The listing builds one solid part. Answer for the finished solid, in the listing's coordinates (mm). Face numbers are marked on the shaded views. Round coordinates to 2 decimals unless told otherwise and drop trailing zeros. Write each loop counter-clockwise with the first axis right and the second up, starting at its lowest first coordinate (ties: lowest second). Pieces come first, ordered by that corner, then holes. Notation, with made-up numbers: (36, 15) - (44, 15) arc R27 cw to (44, 39) - close; hole circle Ø11 at (21, -18). An arc over 180 degrees is marked (long way). Use a Markdown table: item, result. Add a question column.
1) A cutting plane is placed at B-B (x = 63.5). Give the vertices of the cut face in (y, z), then the cut area to 3 significant figures.
2) A cutting plane is placed at D-D (y = 26.5). Give the vertices of the cut face in (x, z), then the cut area to 3 significant figures.
3) A cutting plane is placed at C-C (z = -2). Give the vertices of the cut face in (x, y), then the cut area to 3 significant figures.
4) A cutting plane is placed at A-A (y = 42). Give the vertices of the cut face in (x, z), then the cut area to 3 significant figures.
5) Determine the mould class of the marked faces 1, 2 and 3 for opening direction X: +X half, -X half, draft (parallel to the pull), parting line (faces both ways), or undercut.
6) Find the intervals of material crossed by probe 1 along X at (y, z) = (35, -2.5); probe 2 along X at (y, z) = (13, -5.75); probe 3 along Y at (x, z) = (9.5, -13.5), in increasing order. Write a range as from..to.
7) Each of these flat-tipped pins is pushed along its axis until it touches: P1, Ø6.5, axis at x = 9.5, z = -12.5, coming from the -Y side; P2, Ø5.5, axis at x = 99.5, y = 69, coming from the -Z side; P3, Ø2.5, axis at y = 66, z = -7, coming from the -X side. Where does it stop, or does it pass through?
Autodesk Fusion 360 part; units mm, degrees
sketch "Esquisse1" plane through (0, 0, 0) normal (0, 0, 1) x (1, 0, 0)
  line L0 (102.7, 76) -> (3, 76)
  line L1 (0, 73) -> (0, 3)
  arc A0 (3, 76) -> (0, 73) centre (3, 73) ccw
  arc A1 (0, 3) -> (3, 0) centre (3, 3) ccw
  arc A2 (105.7, 73) -> (102.7, 76) centre (102.7, 73) ccw
  line L2 (6.5, 46.3) -> (12.55, 46.3)
  line L3 (12.55, 46.3) -> (12.55, 29.7)
  line L4 (12.55, 29.7) -> (6.5, 29.7)
  line L5 (6.5, 29.7) -> (6.5, 46.3)
  line L6 (21.9, 22.7) -> (93.7, 22.7)
  line L7 (93.7, 22.7) -> (93.7, 48.7)
  line L8 (93.7, 48.7) -> (21.9, 48.7)
  line L9 (21.9, 48.7) -> (21.9, 22.7)
  line L10 (12.55, 46.3) -> (6.5, 46.3)
  line L11 (6.5, 46.3) -> (6.5, 48.1)
  line L12 (6.5, 48.1) -> (12.55, 48.1)
  line L13 (12.55, 48.1) -> (12.55, 46.3)
  line L14 (12.55, 29.7) -> (6.5, 29.7)
  line L15 (6.5, 29.7) -> (6.5, 27.9)
  line L16 (6.5, 27.9) -> (12.55, 27.9)
  line L17 (12.55, 27.9) -> (12.55, 29.7)
  line L18 (2, 62) -> (1.9999, 62)
  line L19 (105.7, 73) -> (105.7, 3)
  arc A3 (102.7, 0) -> (105.7, 3) centre (102.7, 3) ccw
  line L20 (12.55, 27.9) -> (13.55, 27.9)
  line L21 (13.55, 27.9) -> (13.55, 48.1)
  line L22 (13.55, 48.1) -> (12.55, 48.1)
  line L23 (12.55, 48.1) -> (12.55, 27.9)
  line L24 (2, 14) -> (2, 7)
  line L25 (7, 2) -> (14, 2)
  arc A4 (2, 7) -> (7, 2) centre (7, 7) ccw
  line L26 (2, 14) -> (4, 14)
  line L27 (4, 14) -> (4, 7)
  line L28 (7, 4) -> (14, 4)
  line L29 (14, 2) -> (14, 4)
  arc A5 (4, 7) -> (7, 4) centre (7, 7) ccw
  line L30 (13.67, 2.33) -> (13.67, 3.67)
  line L31 (7, 3.67) -> (13.67, 3.67)
  arc A6 (3.67, 7) -> (7, 3.67) centre (7, 7) ccw
  line L32 (3.67, 13.67) -> (3.67, 7)
  line L33 (2.33, 13.67) -> (3.67, 13.67)
  line L34 (2.33, 13.67) -> (2.33, 7)
  arc A7 (2.33, 7) -> (7, 2.33) centre (7, 7) ccw
  line L35 (7, 2.33) -> (13.67, 2.33)
  line L36 (91.7, 2) -> (98.7, 2)
  line L37 (103.7, 7) -> (103.7, 14)
  line L38 (103.7, 14) -> (101.7, 14)
  line L39 (101.7, 14) -> (101.7, 7)
  line L40 (98.7, 4) -> (91.7, 4)
  line L41 (91.7, 4) -> (91.7, 2)
  arc A8 (98.7, 2) -> (103.7, 7) centre (98.7, 7) ccw
  arc A9 (98.7, 4) -> (101.7, 7) centre (98.7, 7) ccw
  line L42 (92.03, 2.33) -> (98.7, 2.33)
  arc A10 (98.7, 2.33) -> (103.37, 7) centre (98.7, 7) ccw
  line L43 (103.37, 7) -> (103.37, 13.67)
  line L44 (103.37, 13.67) -> (102.03, 13.67)
  line L45 (102.03, 13.67) -> (102.03, 7)
  arc A11 (98.7, 3.67) -> (102.03, 7) centre (98.7, 7) ccw
  line L46 (98.7, 3.67) -> (92.03, 3.67)
  line L47 (92.03, 3.67) -> (92.03, 2.33)
  line L48 (3, 0) -> (102.7, 0)
  line L49 (103.7, 62) -> (103.7, 69)
  line L50 (98.7, 74) -> (91.7, 74)
  line L51 (91.7, 74) -> (91.7, 72)
  line L52 (91.7, 72) -> (98.7, 72)
  line L53 (101.7, 69) -> (101.7, 62)
  line L54 (101.7, 62) -> (103.7, 62)
  arc A12 (101.7, 69) -> (98.7, 72) centre (98.7, 69) ccw
  arc A13 (103.7, 69) -> (98.7, 74) centre (98.7, 69) ccw
  line L55 (92.03, 72.33) -> (98.7, 72.33)
  arc A14 (102.03, 69) -> (98.7, 72.33) centre (98.7, 69) ccw
  line L56 (102.03, 69) -> (102.03, 62.33)
  line L57 (102.03, 62.33) -> (103.37, 62.33)
  line L58 (103.37, 62.33) -> (103.37, 69)
  arc A15 (103.37, 69) -> (98.7, 73.67) centre (98.7, 69) ccw
  line L59 (98.7, 73.67) -> (92.03, 73.67)
  line L60 (92.03, 73.67) -> (92.03, 72.33)
  line L61 (2, 62) -> (2, 69)
  line L62 (7, 74) -> (14, 74)
  line L63 (14, 74) -> (14, 72)
  line L64 (14, 72) -> (7, 72)
  line L65 (4, 69) -> (4, 62)
  line L66 (4, 62) -> (2, 62)
  arc A16 (7, 74) -> (2, 69) centre (7, 69) ccw
  arc A17 (7, 72) -> (4, 69) centre (7, 69) ccw
  line L67 (2.33, 62.33) -> (2.33, 69)
  arc A18 (7, 73.67) -> (2.33, 69) centre (7, 69) ccw
  line L68 (7, 73.67) -> (13.67, 73.67)
  line L69 (13.67, 73.67) -> (13.67, 72.33)
  line L70 (13.67, 72.33) -> (7, 72.33)
  arc A19 (7, 72.33) -> (3.67, 69) centre (7, 69) ccw
  line L71 (3.67, 69) -> (3.67, 62.33)
  line L72 (3.67, 62.33) -> (2.33, 62.33)
  point P0 (0, 76)
  point P1 (103.7, 2)
  point P2 (103.7, 74)
  point P3 (2, 74)
  dimension "d2" = 76
  dimension "d3" = 3
  dimension "d4" = 3
  dimension "d5" = 3
  dimension "d31" = 6.05
  dimension "d32" = 16.6
  dimension "d49" = 26
  dimension "d50" = 71.8
  dimension "d51" = 27.3
  dimension "d53" = 29.7
  dimension "d55" = 1.8
  dimension "d56" = 1.8
  dimension "d72" = 21.9
  dimension "d92" = 6.5
  dimension "d107" = 3
  dimension "d108" = 105.7
  dimension "d109" = 12
  dimension "d137" = 1
  dimension "d147" = 2
  dimension "d148" = 5
  dimension "d149" = 2
  dimension "d150" = 3
  dimension "d151" = 12
  dimension "d152" = 12
  dimension "d153" = -0.33
  dimension "d154" = 12
  dimension "d155" = 12
  dimension "d160" = 2
  dimension "d162" = 2
  dimension "d164" = 5
  dimension "d165" = 3
  dimension "d166" = -0.33
  dimension "d167" = 12
  dimension "d168" = 12
  dimension "d169" = 2
  dimension "d171" = 2
  dimension "d172" = 2
  dimension "d173" = 2
  dimension "d174" = 2
  dimension "d175" = 3
  dimension "d176" = 5
  dimension "d177" = -0.33
  dimension "d178" = 12
  dimension "d179" = 12
  dimension "d180" = 2
  dimension "d183" = 2
  dimension "d184" = 2
  dimension "d185" = 2
  dimension "d186" = 5
  dimension "d187" = 3
  dimension "d188" = -0.33
extrude "Extrusion1" add sketch "Esquisse1" against normal blind 4 contours L0 L1 A0 A1 A2 L19 A3 L48 | L24 L25 A4 L26 L27 L28 L29 A5 | L36 L37 L38 L39 L40 L41 A8 A9 | L49 L50 L51 L52 L53 L54 A12 A13 | L61 L62 L63 L64 L65 L66 A16 A17
extrude "Extrusion5" add sketch "Esquisse1" against normal blind 17 contours L2 L10 L11 L12 L13 L23 | L3 L13 L17 L20 L21 L22 L23 | L4 L14 L15 L16 L17 L23
extrude "Extrusion17" add sketch "Esquisse1" against normal blind 9 contours L30 L31 A6 L32 L33 L34 A7 L35 | L42 A10 L43 L44 L45 A11 L46 L47 | L55 A14 L56 L57 L58 A15 L59 L60 | L67 A18 L68 L69 L70 A19 L71 L72
equation "d36 = 17.55 mm - 3 mm"
equation "d41 = d32 - 0 mm"
equation "d53 = ( d2 - d32 ) / 2"
equation "d56 = d55"
equation "d159 = d158"
equation "d97 = d78"
equation "d98 = d79"
equation "d100 = d81"
equation "d103 = d87"
equation "d104 = d85"
equation "d112 = d80"
equation "d147 = d146"
equation "d152 = d151"
equation "d166 = d153"
equation "d177 = d166"
equation "d188 = d153"
equation "d189 = -4 mm - 5 mm"
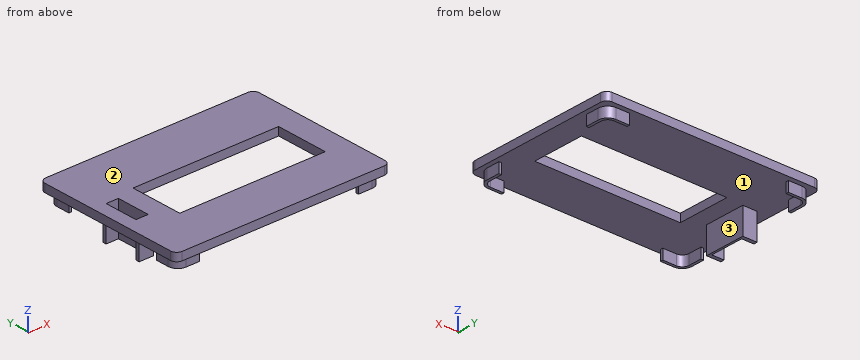
Entries:
| question | item | result |
|---|---|---|
| 1 | outline | (0, -4) - (22.7, -4) - (22.7, 0) - (0, 0) - close; (48.7, -4) - (76, -4) - (76, 0) - (48.7, 0) - close |
| 1 | area | 200 mm² |
| 2 | outline | (0, -4) - (21.9, -4) - (21.9, 0) - (0, 0) - close; (93.7, -4) - (105.7, -4) - (105.7, 0) - (93.7, 0) - close |
| 2 | area | 136 mm² |
| 3 | outline | (0, 3) arc R3 ccw to (3, 0) - (102.7, 0) arc R3 ccw to (105.7, 3) - (105.7, 73) arc R3 ccw to (102.7, 76) - (3, 76) arc R3 ccw to (0, 73) - close; hole (6.5, 29.7) - (12.55, 29.7) - (12.55, 46.3) - (6.5, 46.3) - close; hole (21.9, 22.7) - (93.7, 22.7) - (93.7, 48.7) - (21.9, 48.7) - close |
| 3 | area | 6,060 mm² |
| 4 | outline | (0, -4) - (6.5, -4) - (6.5, 0) - (0, 0) - close; (12.55, -17) - (13.55, -17) - (13.55, -4) - (21.9, -4) - (21.9, 0) - (12.55, 0) - close; (93.7, -4) - (105.7, -4) - (105.7, 0) - (93.7, 0) - close |
| 4 | area | 124 mm² |
| 5 | face 1 | undercut |
| 5 | face 2 | draft |
| 5 | face 3 | +X half |
| 6 | probe 1 | x = 0..6.5, 12.55..21.9, 93.7..105.7 |
| 6 | probe 2 | x = 2.33..3.67, 102.03..103.37 |
| 6 | probe 3 | y = 27.9..29.7, 46.3..48.1 |
| 7 | P1 | stops at y = 27.9 |
| 7 | P2 | stops at z = -9 |
| 7 | P3 | stops at x = 2.33 |
